from build123d import *

# Parameters (mm, degrees)
SKETCH_W        = 140
SKETCH_H        = 70
PAD_DEPTH       = 10
SKETCH001_W     = 140
SKETCH001_H     = 60
POCKET_DEPTH    = 2
FILLET_R        = 1
SKETCH002_W     = 3
SKETCH002_H     = 5
POCKET001_DEPTH = 10.001
FILLET001_R     = 0.5
FILLET002_R     = 0.5


with BuildPart() as part:
    # Sketch → Pad (new body)
    with BuildSketch(Plane.XY):
        with Locations((70, 35)):
            Rectangle(SKETCH_W, SKETCH_H)
    extrude(amount=PAD_DEPTH)

    # Sketch001 (on Face6 of Pad) → Pocket (cut)
    with BuildSketch(Plane.XY.offset(10)):
        with Locations((70, 30)):
            Rectangle(SKETCH001_W, SKETCH001_H)
    extrude(amount=-POCKET_DEPTH, mode=Mode.SUBTRACT)

    # Fillet
    fillet_edges = [part.edges().sort_by_distance(p)[0] for p in [
        (0, 30, 8),
        (70, 0, 8),
        (140, 30, 8),
        (70, 60, 10),
        (140, 65, 10),
        (70, 70, 10),
        (0, 65, 10),
        (0, 60, 9),
        (140, 60, 9),
    ]]
    fillet(fillet_edges, radius=FILLET_R)

    # Sketch002 (on Face10 of Fillet) → Pocket001 (cut, through all)
    with BuildSketch(Plane.XY.offset(10)):
        with Locations((6.5, 65)):
            Rectangle(SKETCH002_W, SKETCH002_H)
        with Locations((21.5, 65)):
            Rectangle(SKETCH002_W, SKETCH002_H)
        with Locations((118.5, 65)):
            Rectangle(SKETCH002_W, SKETCH002_H)
        with Locations((133.5, 65)):
            Rectangle(SKETCH002_W, SKETCH002_H)
    extrude(amount=-POCKET001_DEPTH, mode=Mode.SUBTRACT)

    # Fillet001
    fillet001_edges = [part.edges().sort_by_distance(p)[0] for p in [
        (5, 65, 10),
        (6.5, 67.5, 10),
        (8, 65, 10),
        (6.5, 62.5, 10),
        (21.5, 67.5, 10),
        (20, 65, 10),
        (23, 65, 10),
        (21.5, 62.5, 10),
        (117, 65, 10),
        (118.5, 67.5, 10),
        (120, 65, 10),
        (118.5, 62.5, 10),
        (133.5, 67.5, 10),
        (132, 65, 10),
        (133.5, 62.5, 10),
        (135, 65, 10),
    ]]
    fillet(fillet001_edges, radius=FILLET001_R)

    # Fillet002
    fillet002_edges = [part.edges().sort_by_distance(p)[0] for p in [
        (5, 65, 0),
        (6.5, 62.5, 0),
        (8, 65, 0),
        (6.5, 67.5, 0),
        (21.5, 62.5, 0),
        (20, 65, 0),
        (21.5, 67.5, 0),
        (23, 65, 0),
        (117, 65, 0),
        (118.5, 62.5, 0),
        (120, 65, 0),
        (118.5, 67.5, 0),
        (132, 65, 0),
        (133.5, 62.5, 0),
        (135, 65, 0),
        (133.5, 67.5, 0),
    ]]
    fillet(fillet002_edges, radius=FILLET002_R)


solid = part.part
For this review, take the finished solid that the model builds, in its own axes (mm). A direction names the side the tool comes from. Give positions to 0.01 mm unless a question says otherwise; leave off trailing zeros. Order: outer loops, then holes, each group sorted by start corner. A loop starts at its lowest first (then second) coordinate and runs counter-clockwise, first axis right, second up. Notation, with made-up numbers: M 1,17.5 L 13,17.5 A17 cw 13,24.5 Z; hole C -0.75,32.5 d2. An arc over 180 degrees is marked long. Answer in a Markdown table with one row per item. Add a question column.
(1) Mouldability with a two-part tool opening along X and no side actions: class faces 1 (the face through (118, 67.5, 5)), 2 (the face through (0, 35, 3)), 3 (the face through (20, 65, 5)), 4 (the face through (69, 70, 4)) as +X half, -X half, draft (parallel to the pull), parting line (faces both ways), or undercut.
(2) For pin 1 (6 mm diameter, centred on x = 38.5, y = 9, fed in from +Z), flat-tipped, find the tip position at first contact; note if it passes through.
(3) Consider section B-B on x = 113. State the section outline as (y, z) points.
(4) Wall thickness on probe 1 along X at (y, z) = (63, 8); probe 2 along Y at (x, z) = (22, 1.75); probe 3 along Z at (x, y) = (24, 39.5): over which ranges is each line inside the solid? List them lowest first. Write a range as [from, to].
(5) For faces 5 (the face through (6, 67.5, 5)), 6 (the face through (140, 35, 3)), list the 3-axis set-ups (+Z, -Z, +X, -X, +Y, -Y) from which the entire face can be reached by the end or side of a thin tool; tool diameter is ignored.
(6) Consider section A-A on y = 42. State the section outline as (x, z) points.
Evaluation:
| question | item | result |
|---|---|---|
| 1 | face 1 | undercut |
| 1 | face 2 | -X half |
| 1 | face 3 | undercut |
| 1 | face 4 | draft |
| 2 | pin 1 | stops at z = 8 |
| 3 | outline | M 0,0 L 70,0 L 70,9 A1 ccw 69,10 L 61,10 A1 ccw 60,9 L 60,8 L 1,8 A1 ccw 0,7 Z |
| 4 | probe 1 | x = [0, 5], [8, 20], [23, 117], [120, 132], [135, 140] |
| 4 | probe 2 | y = [0, 62.5], [67.5, 70] |
| 4 | probe 3 | z = [0, 8] |
| 5 | face 5 | +Z, -Z |
| 5 | face 6 | +Z, -Z, +X, +Y, -Y |
| 6 | outline | M 0,0 L 140,0 L 140,7 A1 ccw 139,8 L 1,8 A1 ccw 0,7 Z |
